Autodesk Inventor part; units mm, degrees
ref_plane "YZ Plane" through (0, 0, 0) normal (1, 0, 0) x (0, 1, 0)
ref_plane "XZ Plane" through (0, 0, 0) normal (0, 1, 0) x (-1, 0, 0)
ref_plane "XY Plane" through (0, 0, 0) normal (0, 0, 1) x (1, 0, 0)
sketch "スケッチ1" plane through (0, 0, 0) normal (0, 0, 1) x (1, 0, 0)
  line L0 (0, 0) -> (120, 0)
  line L1 (120, 0) -> (120, 120)
  line L2 (120, 120) -> (0, 120)
  line L3 (0, 120) -> (0, 0)
  dimension "d1" = 120
  dimension "d2" = 120
extrude "押し出し1" add sketch "スケッチ1" along normal blind 1
sketch "スケッチ2" plane through (0, 0, 1) normal (0, 0, 1) x (1, 0, 0)
  line L0 (0, 120) -> (0, 0)
  line L1 (0, 60) -> (120, 60) construction
  line L2 (120, 0) -> (120, 120)
  line L3 (120, 120) -> (0, 120)
  point P0 (13, 115)
  point P1 (13, 90)
  point P2 (43, 115)
  point P3 (43, 90)
  dimension "d8" = 13
  dimension "d9" = 5
  dimension "d12" = 25
  dimension "d15" = 30
hole "穴1" at (13, 115, 1) at (13, 90, 1) at (43, 115, 1) at (43, 90, 1) direction (0, 0, -1) diameter 3.5 end through all
sketch "スケッチ3" plane through (0, 0, 1) normal (0, 0, 1) x (1, 0, 0)
  line L0 (0, 120) -> (0, 0)
  line L1 (0, 0) -> (120, 0)
  point P0 (13, 5)
  point P1 (43, 5)
  point P2 (13, 30)
  point P3 (43, 30)
  dimension "d25" = 13
  dimension "d26" = 5
  dimension "d29" = 30
  dimension "d32" = 25
hole "穴2" at (13, 5, 1) at (43, 5, 1) at (13, 30, 1) at (43, 30, 1) direction (0, 0, -1) diameter 3.5 end through all
sketch "スケッチ4" plane through (0, 0, 1) normal (0, 0, 1) x (1, 0, 0)
  line L0 (0, 120) -> (0, 0)
  line L1 (0, 60) -> (120, 60) construction
  line L2 (120, 0) -> (120, 120)
  line L3 (120, 120) -> (0, 120)
  point P0 (5, 60)
  point P1 (25, 60)
  dimension "d42" = 5
  dimension "d43" = 60
  dimension "d46" = 20
hole "穴3" at (5, 60, 1) at (25, 60, 1) direction (0, 0, -1) diameter 3.5 end through all
sketch "スケッチ5" plane through (0, 0, 1) normal (0, 0, 1) x (1, 0, 0)
  line L0 (0, 120) -> (0, 0)
  line L1 (120, 120) -> (0, 120)
  point P0 (15, 60)
  dimension "d58" = 15
  dimension "d59" = 60
hole "穴4" at (15, 60, 1) direction (0, 0, -1) diameter 10 end through all
sketch "スケッチ6" plane through (0, 0, 1) normal (0, 0, 1) x (1, 0, 0)
  line L0 (0, 120) -> (0, 0)
  line L1 (120, 120) -> (0, 120)
  point P0 (55, 60)
  dimension "d67" = 55
  dimension "d68" = 60
hole "穴5" at (55, 60, 1) direction (0, 0, -1) diameter 12 end through all
sketch "スケッチ7" plane through (0, 0, 1) normal (0, 0, 1) x (1, 0, 0)
  line L0 (0, 120) -> (0, 0)
  line L1 (0, 60) -> (120, 60) construction
  line L2 (120, 0) -> (120, 120)
  line L3 (120, 120) -> (0, 120)
  point P0 (64, 95.25)
  point P1 (64, 24.75)
  point P2 (114.2, 95.25)
  point P3 (114.2, 24.75)
  dimension "d76" = 64
  dimension "d77" = 24.75
  dimension "d80" = 70.5
  dimension "d83" = 50.2
hole "穴6" at (64, 95.25, 1) at (64, 24.75, 1) at (114.2, 95.25, 1) at (114.2, 24.75, 1) direction (0, 0, -1) diameter 3.5 end through all
sketch "スケッチ8" plane through (0, 0, 1) normal (0, 0, 1) x (1, 0, 0)
  line L0 (0, 120) -> (0, 0)
  line L1 (120, 120) -> (0, 120)
  point P0 (85, 72)
  point P1 (85, 48)
  point P2 (115, 72)
  point P3 (115, 48)
  dimension "d93" = 85
  dimension "d94" = 48
  dimension "d97" = 24
  dimension "d100" = 30
hole "穴7" at (85, 72, 1) at (85, 48, 1) at (115, 72, 1) at (115, 48, 1) direction (0, 0, -1) diameter 4.5 end through all
properties part number "RD002"
For this review, take the finished solid that the model builds, in its own axes (mm). Give positions to 0.01 mm unless a question says otherwise; leave off trailing zeros. Write each loop counter-clockwise with the first axis right and the second up, starting at its lowest first coordinate (ties: lowest second). Pieces come first, ordered by that corner, then holes.
Item 1: Wall thickness on probe 1 along X at (y, z) = (95.25, 0.35); probe 2 along X at (y, z) = (48, 0.8); probe 3 along X at (y, z) = (60, 0.6): over which ranges is each line inside the solid? List them lowest first.
Item 2: Take a section at B-B (z = 0.75). Give the number of separate pieces and of enclosed holes in the cut face, and give its area (3 significant figures).
Item 3: Insertion check: P1, Ø3, axis at x = 64, y = 24.75, coming from the -Z side. The pin has a flat end and moves straight along its axis. Give the tip position at first contact, or say it passes through.
Item 4: Take a section at D-D (y = 72). Give the boundary of the cut face in (x, z).
Item 5: Take a section at C-C (x = 5). Give the boundary of the cut face in (y, z), and give its area (4 significant figures).
Item 6: The part is to be moulded in two halves that separate along X. For faces 1 (the face through (72, 61, 1)), 2 (the face through (11.265, 5.228, 0.493)), say which applies: +X half, -X half, draft (parallel to the pull), parting line (faces both ways), or undercut.
Item 7: Take a section at A-A (y = 115). Give the boundary of the cut face in (x, z), and give its area (3 significant figures).
Established:
1. probe 1: x = 0 to 62.25, 65.75 to 112.45, 115.95 to 120
1. probe 2: x = 0 to 82.75, 87.25 to 112.75, 117.25 to 120
1. probe 3: x = 0 to 3.25, 6.75 to 10, 20 to 23.25, 26.75 to 49, 61 to 120
2. separate pieces: 1
2. enclosed holes: 20
2. area: 14,000 mm2
3. P1: passes through
4. outline: (0, 0) - (82.75, 0) - (82.75, 1) - (0, 1) - close; (87.25, 0) - (112.75, 0) - (112.75, 1) - (87.25, 1) - close; (117.25, 0) - (120, 0) - (120, 1) - (117.25, 1) - close
5. outline: (0, 0) - (58.25, 0) - (58.25, 1) - (0, 1) - close; (61.75, 0) - (120, 0) - (120, 1) - (61.75, 1) - close
5. area: 116.5 mm2
6. face 1: draft
6. face 2: undercut
7. outline: (0, 0) - (11.25, 0) - (11.25, 1) - (0, 1) - close; (14.75, 0) - (41.25, 0) - (41.25, 1) - (14.75, 1) - close; (44.75, 0) - (120, 0) - (120, 1) - (44.75, 1) - close
7. area: 113 mm2
